CAD build for the part. Positions are in the model's coordinates, mm. Face numbers are marked on the shaded views. Round coordinates to 2 decimals unless told otherwise and drop trailing zeros. Loops run counter-clockwise (first coordinate to the right, second up) from the corner with the lowest first, then second, coordinate; pieces in that order, holes last.
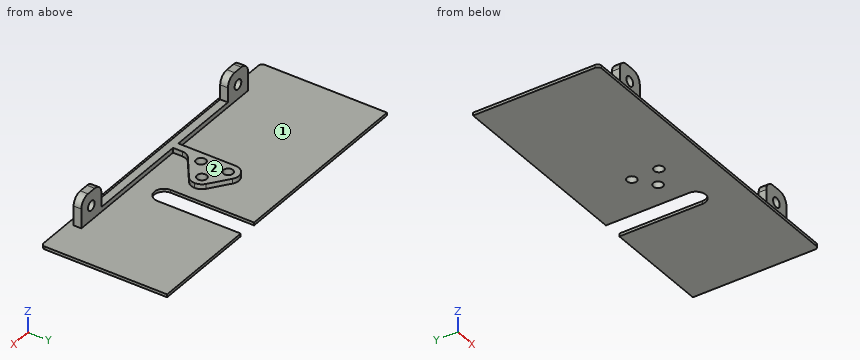
from build123d import *

# Parameters (mm, degrees)
F2_DEPTH  = 1.5
F1_W      = 15
F1_H      = 4
F3_DEPTH  = 16.5
F1_R      = 2.5
F4_DEPTH  = 4
F5_R      = 2.5
F6_DEPTH  = 62.001
F7_R      = 5
F10_ANGLE = 180


with BuildPart() as f2:
    # F1 (on Top) → F2 (new body)
    with BuildSketch(Plane.XY):
        with BuildLine():
            Line((-82.5, 63), (-82.5, 0))
            Line((-82.5, 0), (17.25, 0))
            Line((17.25, 0), (17.25, 43))
            ThreePointArc((17.25, 43), (22.25, 48), (27.25, 43))
            Line((27.25, 43), (27.25, 0))
            Line((27.25, 0), (82.5, 0))
            Line((82.5, 0), (82.5, 63))
            ThreePointArc((82.5, 63), (81.9142135624, 64.4142135624), (80.5, 65))
            Line((80.5, 65), (-80.5, 65))
            ThreePointArc((-80.5, 65), (-81.9142135624, 64.4142135624), (-82.5, 63))
        make_face()
        with BuildLine():
            Line((-62.5, 58), (-62.5, 62))
            Line((-62.5, 62), (-47.5, 62))
            Line((-47.5, 62), (47.5, 62))
            Line((47.5, 62), (62.5, 62))
            Line((62.5, 62), (62.5, 58))
            Line((62.5, 58), (47.5, 58))
            Line((47.5, 58), (-6.25, 58))
            Line((-6.25, 58), (-6.25, 53.2162800982))
            ThreePointArc((-6.25, 53.2162800982), (-5.6588833201, 50.735783263), (-4.0125947093, 48.7884729928))
            Line((-4.0125947093, 48.7884729928), (8.0125947093, 39.9278071054))
            ThreePointArc((8.0125947093, 39.9278071054), (9.6588833201, 37.9804968352), (10.25, 35.5))
            ThreePointArc((10.25, 35.5), (9.6588833201, 33.0195031648), (8.0125947093, 31.0721928946))
            Line((8.0125947093, 31.0721928946), (-1.4874052907, 24.0721928946))
            ThreePointArc((-1.4874052907, 24.0721928946), (-7.2304968352, 23.5911166799), (-10.25, 28.5))
            Line((-10.25, 28.5), (-10.25, 58))
            Line((-10.25, 58), (-47.5, 58))
            Line((-47.5, 58), (-62.5, 58))
        make_face(mode=Mode.SUBTRACT)
    extrude(amount=F2_DEPTH)

    # F1 (on Top) → F3 (join)
    with BuildSketch(Plane.XY):
        with Locations((-55, 60)):
            Rectangle(F1_W, F1_H)
        with Locations((55, 60)):
            Rectangle(F1_W, F1_H)
    extrude(amount=F3_DEPTH)

    # F1 (on Top) → F4 (join)
    with BuildSketch(Plane.XY):
        Polygon((47.5, 62), (-47.5, 62), (-47.5, 58), (-10.25, 58), (-6.25, 58), (47.5, 58), align=None)
        with BuildLine():
            Line((-6.25, 58), (-10.25, 58))
            Line((-10.25, 58), (-10.25, 28.5))
            ThreePointArc((-10.25, 28.5), (-7.2304968352, 23.5911166799), (-1.4874052907, 24.0721928946))
            Line((-1.4874052907, 24.0721928946), (8.0125947093, 31.0721928946))
            ThreePointArc((8.0125947093, 31.0721928946), (9.6588833201, 33.0195031648), (10.25, 35.5))
            ThreePointArc((10.25, 35.5), (9.6588833201, 37.9804968352), (8.0125947093, 39.9278071054))
            Line((8.0125947093, 39.9278071054), (-4.0125947093, 48.7884729928))
            ThreePointArc((-4.0125947093, 48.7884729928), (-5.6588833201, 50.735783263), (-6.25, 53.2162800982))
            Line((-6.25, 53.2162800982), (-6.25, 58))
        make_face()
        with Locations((-4.75, 28.5)):
            Circle(F1_R, mode=Mode.SUBTRACT)
        with Locations((-4.75, 42.5)):
            Circle(F1_R, mode=Mode.SUBTRACT)
        with Locations((4.75, 35.5)):
            Circle(F1_R, mode=Mode.SUBTRACT)
    extrude(amount=F4_DEPTH)

    # F5 (on face) → F6 (cut, through all)
    with BuildSketch(Plane(origin=(0, 62, 0), x_dir=(-1, 0, 0), z_dir=(0, 1, 0))):
        with Locations((55, 9)):
            Circle(F5_R)
        with Locations((-55, 9)):
            Circle(F5_R)
    extrude(amount=-F6_DEPTH, mode=Mode.SUBTRACT)

    # F7
    f7_edges = [f2.edges().sort_by_distance(p)[0] for p in [
        (-62.5, 60, 16.5),
        (-47.5, 60, 16.5),
        (47.5, 60, 16.5),
        (62.5, 60, 16.5),
    ]]
    fillet(f7_edges, radius=F7_R)


with BuildPart() as f8_1:
    # F8: instance of F2
    add(f2.part.mirror(Plane.XY))


with BuildPart() as f8_1_1:
    # F10: moved
    add(f8_1.part.rotate(Axis((-32.625, 0, 0), (1, 0, 0)), F10_ANGLE))


solid = f8_1_1.part
Item 1: Mould opens along X. For the marked faces 1 and 2 say: released by +X, released by -X, zero draft, split by the parting line, or undercut.
Verdict:
face 1: zero draft
face 2: undercut
Item 2: Cut at A-A (z = 14.5). List the corners of the cut face in (x, y).
Verdict:
outline: (-61.5, -62) - (-48.5, -62) - (-48.5, -58) - (-61.5, -58) - close; (48.5, -62) - (61.5, -62) - (61.5, -58) - (48.5, -58) - close
Item 3: Wall check: L1, parallel to Y at x = 4.75, z = 1.35; L2, parallel to Y at x = -4.75, z = 2.25; L3, parallel to X at y = -35.5, z = 2.95. Give the ranges that are in metal, low to high.
Verdict:
L1: y = -65 to -38, -33 to 0
L2: y = -62 to -58, -49.44 to -45, -40 to -31, -26 to -23
L3: x = -10.25 to 2.25, 7.25 to 10.25
Item 4: Cut at D-D (y = -56). List the corners of the cut face in (x, z).
Verdict:
outline: (-82.5, 0) - (82.5, 0) - (82.5, 1.5) - (-6.25, 1.5) - (-6.25, 4) - (-10.25, 4) - (-10.25, 1.5) - (-82.5, 1.5) - close
Item 5: Cut at B-B (x = 55). List the corners of the cut face in (y, z).
Verdict:
outline: (-65, 0) - (0, 0) - (0, 1.5) - (-58, 1.5) - (-58, 6.5) - (-62, 6.5) - (-62, 1.5) - (-65, 1.5) - close; (-62, 11.5) - (-58, 11.5) - (-58, 16.5) - (-62, 16.5) - close
Item 6: Cut at C-C (y = -5). List the corners of the cut face in (x, z), plus the area to 4 significant figures.
Verdict:
outline: (-82.5, 0) - (17.25, 0) - (17.25, 1.5) - (-82.5, 1.5) - close; (27.25, 0) - (82.5, 0) - (82.5, 1.5) - (27.25, 1.5) - close
area: 232.5 mm2
Item 7: Flat gauge pins, fed straight in: P1, Ø6.5, axis at x = -4.75, y = -42.5, coming from the -Z side; P2, Ø6.5, axis at x = -55, z = 9, coming from the +Y side; P3, Ø3, axis at y = -59.5, z = 8, coming from the -X side; P4, Ø2, axis at y = -60, z = 8, coming from the +X side. Where does each tip first touch, or does it go through?
Verdict:
P1: stops at z = 0
P2: stops at y = -58
P3: stops at x = -62.5
P4: stops at x = 62.5
